The listing builds one solid part. Answer for the finished solid, in the listing's coordinates (mm). Round coordinates to 2 decimals unless told otherwise and drop trailing zeros. Order: outer loops, then holes, each group sorted by start corner. A loop starts at its lowest first (then second) coordinate and runs counter-clockwise, first axis right, second up. Notation, with made-up numbers: (33, -24) -> (87, -24) arc R21 ccw to (87, 2) -> close; hole circle Ø3 at (29.5, 26). An arc over 180 degrees is marked (long way). Return JSON: item names as keys, results as strings. Group by question number.
(1) Determine the mould class of faces 1 (the face through (19, 0, 82)), 2 (the face through (47.22, 1.61, -37.2)), 3 (the face through (44.737, 1.61, 201.007)), 4 (the face through (-27.08, 1.61, -39.13)) for opening direction Z: +Z half, -Z half, draft (parallel to the pull), parting line (faces both ways), or undercut.
(2) Consider line 1 (X direction, y = 0.25, z = 42.5); line 2 (Z direction, x = 3, y = 0.1); line 3 (X direction, y = 1.4, z = 169.5). Determine where each line is inside the solid, lowest interval first. Write a range as [from, to].
(3) The part is cut by section B-B (y = 1.55). Count the separate pieces of the cut face and the enclosed holes in it, plus the area to 3 significant figures.
(4) The part is cut by section A-A (z = 34). Determine the outline of the cut face in (x, y) (3 decimals).
(5) The part is cut by section C-C (z = 122.5). Determine the outline of the cut face in (x, y) (3 decimals), plus the area to 3 significant figures.
from build123d import *

# Parameters (mm, degrees)
SKETCH1_W           = 101.6
SKETCH1_H           = 254
BOSS_EXTRUDE1_DEPTH = 3.175
SKETCH2_R           = 2.54
SKETCH2_R_2         = 1.25000004
SKETCH2_R_3         = 1.524
CUT_EXTRUDE1_DEPTH  = 223.663234681
FILLET1_R           = 12.7
CUT_EXTRUDE7_DEPTH  = 223.663234681


with BuildPart() as part:
    # Sketch1 → Boss-Extrude1 (new body)
    with BuildSketch(Plane(origin=(0, 0, 0), x_dir=(1, 0, 0), z_dir=(0, 1, 0))):
        with Locations((20.100372359, -84.049692378)):
            Rectangle(SKETCH1_W, SKETCH1_H)
    extrude(amount=BOSS_EXTRUDE1_DEPTH)

    # Sketch2 → Cut-Extrude1 (cut, through all)
    with BuildSketch(Plane(origin=(0, 3.175, 0), x_dir=(1, 0, 0), z_dir=(0, 1, 0))):
        with Locations(Location((-5.299627641, 35.330307622, 0), (0, 0, 270))):
            Circle(SKETCH2_R)
        with Locations(Location((20.100372359, 35.330307622, 0), (0, 0, 270))):
            Circle(SKETCH2_R)
        with Locations(Location((45.500372359, 35.330307622, 0), (0, 0, 270))):
            Circle(SKETCH2_R)
        with Locations(Location((-23.079627641, -84.049692378, 0), (0, 0, 270))):
            Circle(SKETCH2_R)
        with Locations(Location((-23.079627641, -45.949692378, 0), (0, 0, 270))):
            Circle(SKETCH2_R)
        with Locations(Location((-23.079627641, -7.849692378, 0), (0, 0, 270))):
            Circle(SKETCH2_R)
        with Locations(Location((63.280372359, -7.849692378, 0), (0, 0, 90))):
            Circle(SKETCH2_R)
        with Locations(Location((63.280372359, -45.949692378, 0), (0, 0, 90))):
            Circle(SKETCH2_R)
        with Locations(Location((63.280372359, -84.049692378, 0), (0, 0, 90))):
            Circle(SKETCH2_R)
        with Locations(Location((63.280372359, -122.149692378, 0), (0, 0, 270))):
            Circle(SKETCH2_R)
        with Locations(Location((63.280372359, -160.249692378, 0), (0, 0, 270))):
            Circle(SKETCH2_R)
        with Locations(Location((-23.079627641, -160.249692378, 0), (0, 0, 90))):
            Circle(SKETCH2_R)
        with Locations(Location((-23.079627641, -122.149692378, 0), (0, 0, 90))):
            Circle(SKETCH2_R)
        with Locations(Location((45.500372359, -203.429692378, 0), (0, 0, 90))):
            Circle(SKETCH2_R)
        with Locations(Location((20.100372359, -203.429692378, 0), (0, 0, 90))):
            Circle(SKETCH2_R)
        with Locations(Location((-5.299627641, -203.429692378, 0), (0, 0, 90))):
            Circle(SKETCH2_R)
        with Locations(Location((2.955372359, -84.049692378, 0), (0, 0, 270))):
            Circle(SKETCH2_R_2)
        with Locations(Location((37.245372359, -84.049692378, 0), (0, 0, 90))):
            Circle(SKETCH2_R_2)
        with Locations(Location((37.245372359, -169.139692378, 0), (0, 0, 270))):
            Circle(SKETCH2_R_2)
        with Locations(Location((2.955372359, -169.139692378, 0), (0, 0, 90))):
            Circle(SKETCH2_R_2)
        with Locations(Location((-19.399627381, 28.542449069, 0), (0, 0, 270))):
            Circle(SKETCH2_R_3)
        with Locations(Location((59.600372099, 28.542449069, 0), (0, 0, 90))):
            Circle(SKETCH2_R_3)
        with Locations(Location((59.600372099, -13.457550751, 0), (0, 0, 270))):
            Circle(SKETCH2_R_3)
        with Locations(Location((-19.399627381, -13.457550751, 0), (0, 0, 90))):
            Circle(SKETCH2_R_3)
    extrude(amount=-CUT_EXTRUDE1_DEPTH, mode=Mode.SUBTRACT)

    # Fillet1
    fillet1_edges = [part.edges().sort_by_distance(p)[0] for p in [
        (-30.699627641, 1.5875, -42.950307622),
        (70.900372359, 1.5875, -42.950307622),
        (70.900372359, 1.5875, 211.049692378),
        (-30.699627641, 1.5875, 211.049692378),
    ]]
    fillet(fillet1_edges, radius=FILLET1_R)

    # Sketch4 → Cut-Extrude7 (cut, through all)
    with BuildSketch(Plane(origin=(0, 0, 0), x_dir=(1, 0, 0), z_dir=(0, 1, 0))):
        with BuildLine():
            Line((51.42781247, -4.28096808), (51.42781247, -62.218416676))
            ThreePointArc((51.42781247, -62.218416676), (48.25281247, -65.393416676), (45.07781247, -62.218416676))
            Line((45.07781247, -62.218416676), (45.07781247, -4.28096808))
            ThreePointArc((45.07781247, -4.28096808), (48.25281247, -1.10596808), (51.42781247, -4.28096808))
        make_face()
        with BuildLine():
            Line((-10.80218753, -4.28096808), (-10.80218753, -62.218416676))
            ThreePointArc((-10.80218753, -62.218416676), (-7.62718753, -65.393416676), (-4.45218753, -62.218416676))
            Line((-4.45218753, -62.218416676), (-4.45218753, -4.28096808))
            ThreePointArc((-4.45218753, -4.28096808), (-7.62718753, -1.10596808), (-10.80218753, -4.28096808))
        make_face()
    extrude(amount=CUT_EXTRUDE7_DEPTH, mode=Mode.SUBTRACT)


solid = part.part
Answer below:
{
 "1": {"face 1": "draft", "face 2": "undercut", "face 3": "undercut", "face 4": "-Z half"},
 "2": {"line 1": "x = [-30.7, -10.8], [-4.45, 45.08], [51.43, 70.9]", "line 2": "z = [-42.95, 82.8], [85.3, 167.89], [170.39, 211.05]", "line 3": "x = [-30.7, 1.76], [4.15, 36.05], [38.44, 70.9]"},
 "3": {"separate pieces": "1", "enclosed holes": "26", "area": "24,500 mm²"},
 "4": {"outline": "(-30.7, 0) -> (-10.802, 0) -> (-10.802, 3.175) -> (-30.7, 3.175) -> close; (-4.452, 0) -> (45.078, 0) -> (45.078, 3.175) -> (-4.452, 3.175) -> close; (51.428, 0) -> (70.9, 0) -> (70.9, 3.175) -> (51.428, 3.175) -> close"},
 "5": {"outline": "(-30.7, 0) -> (-25.595, 0) -> (-25.595, 3.175) -> (-30.7, 3.175) -> close; (-20.564, 0) -> (60.765, 0) -> (60.765, 3.175) -> (-20.564, 3.175) -> close; (65.796, 0) -> (70.9, 0) -> (70.9, 3.175) -> (65.796, 3.175) -> close", "area": "291 mm²"}
}
